Study the drawing (mm; zero at the part's minimum x, y, z) and answer. A direction names the side the tool comes from. Coordinates: 2 decimals unless noted, no trailing zeros. Loops run counter-clockwise (first coordinate to the right, second up) from the corner with the lowest first, then second, coordinate; pieces in that order, holes last. Notation, with made-up numbers: (66.25, -27) -> (77.25, -27) arc R20 cw to (77.25, 12) -> close; hole circle Ø8 at (17.5, 18). An arc over 180 degrees is marked (long way). Answer in a Markdown table with one row per item.
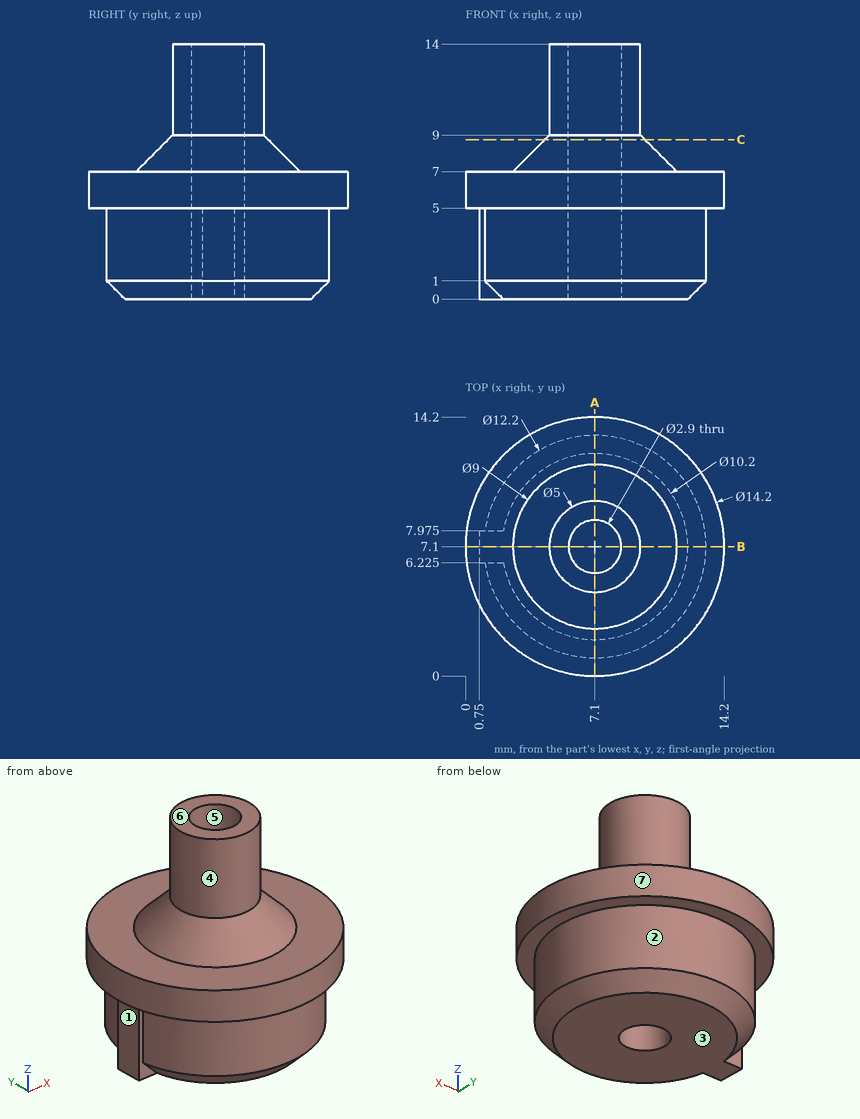
1. A cutting plane is placed at B-B on y = 7.1. Give the vertices of the cut face in (x, z).
A:
| item | result |
|---|---|
| outline | (0, 5) -> (0.75, 5) -> (0.75, 0) -> (5.65, 0) -> (5.65, 14) -> (4.6, 14) -> (4.6, 9) -> (2.6, 7) -> (0, 7) -> close; (8.55, 0) -> (12.2, 0) -> (13.2, 1) -> (13.2, 5) -> (14.2, 5) -> (14.2, 7) -> (11.6, 7) -> (9.6, 9) -> (9.6, 14) -> (8.55, 14) -> close |
2. A tool of negligible diameter and unlimited length cuts with its end or side. For the marked faces 1, 2, 3 and 4, from which of +Z, -Z, +X, -X, +Y, -Y can it reach the whole face along a straight path? Write none if from no direction.
A:
| item | result |
|---|---|
| face 1 | -Z, -X, +Y, -Y |
| face 2 | -Z |
| face 3 | -Z, +X, -X, +Y, -Y |
| face 4 | +Z |
3. Given pin 1 Ø3 at (x, z) = (11.5, 9.5) entering from -Y; pin 2 Ø4 at (x, z) = (2, 1.5) entering from +Y; pin 3 Ø1.5 at (x, z) = (1.5, 1.5) entering from +Y; pin 4 Ø0.5 at (y, z) = (7.5, 1.5) entering from -X, each flat-ended and moving along its own axis, determine where each tip first touches the part or whether it passes through.
A:
| item | result |
|---|---|
| pin 1 | passes through |
| pin 2 | stops at y = 12.35 |
| pin 3 | stops at y = 10.8 |
| pin 4 | stops at x = 0.75 |
4. Find the intervals of material crossed by probe 1 along Y at (x, z) = (7.1, 6.75); probe 2 along X at (y, z) = (6.75, 12.75); probe 3 along Y at (x, z) = (7.5, 2.25), in increasing order.
A:
| item | result |
|---|---|
| probe 1 | y = 0 to 5.65, 8.55 to 14.2 |
| probe 2 | x = 4.62 to 5.69, 8.51 to 9.58 |
| probe 3 | y = 1.01 to 5.71, 8.49 to 13.19 |
5. A cutting plane is placed at A-A on x = 7.1. Give the vertices of the cut face in (y, z), and give its area (3 significant figures).
A:
| item | result |
|---|---|
| outline | (0, 5) -> (1, 5) -> (1, 1) -> (2, 0) -> (5.65, 0) -> (5.65, 14) -> (4.6, 14) -> (4.6, 9) -> (2.6, 7) -> (0, 7) -> close; (8.55, 0) -> (12.2, 0) -> (13.2, 1) -> (13.2, 5) -> (14.2, 5) -> (14.2, 7) -> (11.6, 7) -> (9.6, 9) -> (9.6, 14) -> (8.55, 14) -> close |
| area | 86.8 mm2 |
6. A cutting plane is placed at C-C on z = 8.75. Give the vertices of the cut face in (x, y), and give its area (3 significant figures).
A:
| item | result |
|---|---|
| outline | circle Ø5.5 at (7.1, 7.1); hole circle Ø2.9 at (7.1, 7.1) |
| area | 17.2 mm2 |
7. The mould has two halves that part along Y. Classify the marked faces 5, 6 and 7: pulls with the +Y half, pulls with the -Y half, needs draft (parallel to the pull), parting line crosses it, or undercut.
A:
| item | result |
|---|---|
| face 5 | undercut |
| face 6 | needs draft |
| face 7 | parting line crosses it |
